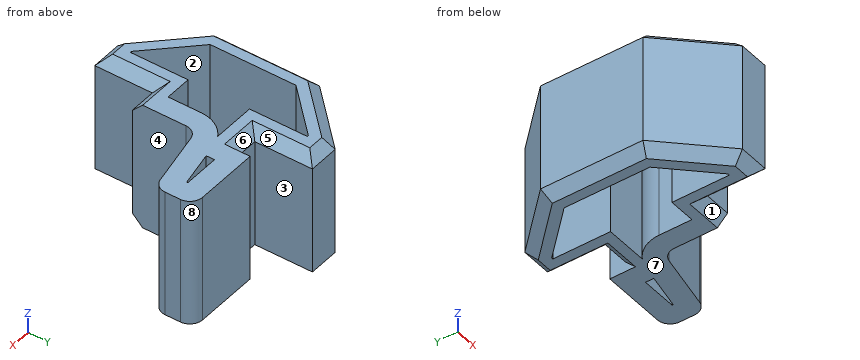
```python
from build123d import *

# Parameters (mm, degrees)
SALIENTE_EXTRUIR1_DEPTH = 5
SALIENTE_EXTRUIR2_DEPTH = 10
REDONDEO1_R             = 1
VACIADO1_START          = -5
VACIADO1_DEPTH          = 10
CHAFL_N1_SIZE           = 0.8


# Read off the part's stored shape, not the designer's step: Vaciado1
with BuildPart() as part:
    # Croquis1 → Saliente-Extruir1 (new, symmetric)
    with BuildSketch(Plane.XY):
        Polygon((0, 4), (-2.1, 4), (-2.1, 8.5), (-4.5, 8.5), (-8.9, 4), (-8.9, -4), (-4.5, -8.5), (-2.1, -8.5), (-2.1, -4), (0, -4), align=None)
    extrude(amount=SALIENTE_EXTRUIR1_DEPTH, both=True)

    # Croquis2 → Saliente-Extruir2 (add, through all)
    with BuildSketch(Plane(origin=(0, 0, -5), x_dir=(-1, 0, 0), z_dir=(0, 0, -1))):
        Polygon((0, 4), (0, 5.2), (-6, 5.2), (-6, 2.2), (0, 1), align=None)
    extrude(amount=-SALIENTE_EXTRUIR2_DEPTH)

    # Redondeo1
    redondeo1_edges = [part.edges().sort_by_distance(p)[0] for p in [
        (0, 1, 0),
        (6, 2.2, 0),
        (6, 5.2, 0),
    ]]
    fillet(redondeo1_edges, radius=REDONDEO1_R)

    # Vaciado1 outline → Vaciado1 (cut)
    with BuildSketch(Plane.XY.offset(VACIADO1_START)):
        Polygon((4.4, 3.511686244), (4.4, 3.6), (1.6, 3.6), (1.6, 2.951686244), align=None)
        with BuildLine():
            Line((-1.6, -2.4), (-1.6, 0.180196097))
            ThreePointArc((-1.6, 0.180196097), (-1.267111406, 1.453069175), (-0.35368779, 2.4))
            Line((-0.35368779, 2.4), (-3.7, 2.4))
            Line((-3.7, 2.4), (-3.7, 6.9))
            Line((-3.7, 6.9), (-3.826703079, 6.9))
            Line((-3.826703079, 6.9), (-7.3, 3.347764512))
            Line((-7.3, 3.347764512), (-7.3, -3.347764512))
            Line((-7.3, -3.347764512), (-3.826703079, -6.9))
            Line((-3.826703079, -6.9), (-3.7, -6.9))
            Line((-3.7, -6.9), (-3.7, -2.4))
            Line((-3.7, -2.4), (-1.6, -2.4))
        make_face()
    extrude(amount=VACIADO1_DEPTH, mode=Mode.SUBTRACT)

    # Chaflán1
    chafl_n1_edges = [part.edges().sort_by_distance(p)[0] for p in [
        (-1.05, -4, -5),
        (-2.1, -6.25, -5),
        (-3.3, -8.5, -5),
        (-6.7, -6.25, -5),
        (-8.9, 0, -5),
        (-6.7, 6.25, -5),
        (-3.3, 8.5, -5),
        (-2.1, 6.25, 5),
        (-2.1, 6.25, -5),
        (-1.05, 4, -5),
        (-3.3, 8.5, 5),
        (-6.7, 6.25, 5),
        (-8.9, 0, 5),
        (-6.7, -6.25, 5),
        (-3.3, -8.5, 5),
        (-2.1, -6.25, 5),
        (-1.05, -4, 5),
        (-1.05, 4, 5),
    ]]
    chamfer(chafl_n1_edges, length=CHAFL_N1_SIZE)


solid = part.part
```
The model under review builds one solid part; all positions refer to its coordinate system, in mm. Face numbers are marked on the shaded views. A direction names the side the tool comes from. Coordinates: 2 decimals unless noted, no trailing zeros. Write each loop counter-clockwise with the first axis right and the second up, starting at its lowest first coordinate (ties: lowest second). Pieces come first, ordered by that corner, then holes.
1) The part is to be moulded in two halves that separate along X. For the marked faces 6, 7 and 8, say which applies: pulls with the +X half, pulls with the -X half, needs draft (parallel to the pull), parting line crosses it, or undercut.
2) We need section A-A on y = -0.75. State the section outline as (x, z) points.
3) Machinability: for the marked faces 1, 2, 3, 4 and 5, which of the approach directions +Z, -Z, +X, -X, +Y, -Y give a long, thin tool a straight path to every point of the face, cutting with its end or side? Answer none if there is none.
4) We need section D-D on y = 5. State the section outline as (x, z) points, then the cut area to 3 significant figures.
5) We need section C-C on z = -1. Count the separate pieces of the cut face and the enclosed holes in it, then the cut area to 3 significant figures.
6) We need section B-B on x = -5.5. State the section outline as (y, z) points, then the cut area to 3 significant figures.
7) To check wall thickness, follow probe 1 along Y at (x, z) = (-2, 0.5); probe 2 along Y at (x, z) = (-3.5, 3); probe 3 along X at (y, z) = (0, -0.25). State the ranges of each line that lie inside material, in increasing order.
8) Clearance check with flat-ended pins moving along their axes: pin 1 Ø5.5 at (x, z) = (1.5, -1) entering from +Y; pin 2 Ø1 at (x, z) = (-1.5, 2) entering from +Y; pin 3 Ø2 at (x, z) = (3.5, 1.5) entering from -Y; pin 4 Ø4 at (y, z) = (2, 3.5) entering from +X. State where each tip first meets the part, or that it passes through.
Answer list:
1. face 6: undercut
1. face 7: needs draft
1. face 8: pulls with the +X half
2. outline: (-8.9, -4.2) - (-8.1, -5) - (-7.3, -5) - (-7.3, 5) - (-8.1, 5) - (-8.9, 4.2) - close; (-1.6, -5) - (0, -5) - (0, 5) - (-1.6, 5) - close
3. face 1: -Z, +X, -Y
3. face 2: +Z, -Z
3. face 3: +Z, -Z, +Y
3. face 4: +Z, -Z, +X, -Y
3. face 5: +Z, +Y
4. outline: (-7.92, -4.2) - (-6.8, -5) - (-5.68, -5) - (-5.68, 5) - (-6.8, 5) - (-7.92, 4.2) - close; (-3.7, -5) - (-2.9, -5) - (-2.1, -4.2) - (-2.1, 4.2) - (-2.9, 5) - (-3.7, 5) - close; (0, -5) - (5.6, -5) - (5.6, 5) - (0, 5) - close
4. area: 92.8 mm2
5. separate pieces: 1
5. enclosed holes: 2
5. area: 84.7 mm2
6. outline: (-7.48, -4.2) - (-6.33, -5) - (-5.19, -5) - (-5.19, 5) - (-6.33, 5) - (-7.48, 4.2) - close; (5.19, -5) - (6.33, -5) - (7.48, -4.2) - (7.48, 4.2) - (6.33, 5) - (5.19, 5) - close
6. area: 43.9 mm2
7. probe 1: y = -4 to -2.4, 2.4 to 4
7. probe 2: y = -8.5 to -2.4, 2.4 to 8.5
7. probe 3: x = -8.9 to -7.3, -1.6 to 0
8. pin 1: stops at y = 5.2
8. pin 2: stops at y = 4
8. pin 3: stops at y = 1.5
8. pin 4: stops at x = 6
